```python
from build123d import *

# Parameters (mm, degrees)
SZKIC1_W                    = 140
SZKIC1_H                    = 70
DODANIE_WYCI_GNI_CIE1_DEPTH = 5
SZKIC2_W                    = 4
SZKIC2_H                    = 30
DODANIE_WYCI_GNI_CIE2_DEPTH = 25
SZKIC3_W                    = 10
SZKIC3_H                    = 30
SZKIC3_W_2                  = 2
DODANIE_WYCI_GNI_CIE3_DEPTH = 2
SZKIC4_R                    = 0.75
WYTNIJ_WYCI_GNI_CIE1_DEPTH  = 12
WYTNIJ_WYCI_GNI_CIE2_START  = -12
SZKIC5_R                    = 0.75
WYTNIJ_WYCI_GNI_CIE2_DEPTH  = 12
SZKIC6_W                    = 5
SZKIC6_H                    = 20
WYTNIJ_WYCI_GNI_CIE3_DEPTH  = 12
SZKIC8_R                    = 1
WYTNIJ_WYCI_GNI_CIE4_DEPTH  = 12


with BuildPart() as part:
    # Szkic1 → Dodanie-wyciągnięcie1 (new body)
    with BuildSketch(Plane(origin=(0, 0, 0), x_dir=(1, 0, 0), z_dir=(0, 1, 0))):
        with Locations((70, -35)):
            Rectangle(SZKIC1_W, SZKIC1_H)
    extrude(amount=DODANIE_WYCI_GNI_CIE1_DEPTH)

    # Szkic2 → Dodanie-wyciągnięcie2 (add)
    with BuildSketch(Plane.XZ):
        with Locations((2, 35)):
            Rectangle(SZKIC2_W, SZKIC2_H)
        with Locations((138, 35)):
            Rectangle(SZKIC2_W, SZKIC2_H)
        with Locations((70, 35)):
            Rectangle(SZKIC2_W, SZKIC2_H)
    extrude(amount=DODANIE_WYCI_GNI_CIE2_DEPTH)

    # Szkic3 → Dodanie-wyciągnięcie3 (add)
    with BuildSketch(Plane.XZ.offset(25)):
        with Locations((77, 35)):
            Rectangle(SZKIC3_W, SZKIC3_H)
        with Locations((63, 35)):
            Rectangle(SZKIC3_W, SZKIC3_H)
        with Locations((71, 35)):
            Rectangle(SZKIC3_W_2, SZKIC3_H)
        with Locations((69, 35)):
            Rectangle(SZKIC3_W_2, SZKIC3_H)
    extrude(amount=DODANIE_WYCI_GNI_CIE3_DEPTH)

    # Szkic4 → Wytnij-wyciągnięcie1 (cut)
    with BuildSketch(Plane.ZY):
        with Locations((35, -2.75)):
            Circle(SZKIC4_R)
        with Locations((35, -21.25)):
            Circle(SZKIC4_R)
    extrude(amount=-WYTNIJ_WYCI_GNI_CIE1_DEPTH, mode=Mode.SUBTRACT)

    # Szkic5 → Wytnij-wyciągnięcie2 (cut)
    with BuildSketch(Plane(origin=(140, 0, 0), x_dir=(0, 0, -1), z_dir=(1, 0, 0)).offset(WYTNIJ_WYCI_GNI_CIE2_START)):
        with Locations(Location((-35, -21.25, 0), (0, 0, 180))):
            Circle(SZKIC5_R)
        with Locations(Location((-35, -2.75, 0), (0, 0, 180))):
            Circle(SZKIC5_R)
    extrude(amount=WYTNIJ_WYCI_GNI_CIE2_DEPTH, mode=Mode.SUBTRACT)

    # Szkic6 → Wytnij-wyciągnięcie3 (cut)
    with BuildSketch(Plane(origin=(0, 5, 0), x_dir=(1, 0, 0), z_dir=(0, 1, 0))):
        with Locations((58.5, -35)):
            Rectangle(SZKIC6_W, SZKIC6_H)
        with Locations((81.5, -35)):
            Rectangle(SZKIC6_W, SZKIC6_H)
    extrude(amount=-WYTNIJ_WYCI_GNI_CIE3_DEPTH, mode=Mode.SUBTRACT)

    # Szkic8 → Wytnij-wyciągnięcie4 (cut)
    with BuildSketch(Plane(origin=(0, 5, 0), x_dir=(1, 0, 0), z_dir=(0, 1, 0))):
        with Locations(Location((135, -65, 0), (0, 0, 270))):
            Circle(SZKIC8_R)
        with Locations(Location((135, -5, 0), (0, 0, 270))):
            Circle(SZKIC8_R)
        with Locations(Location((5, -5, 0), (0, 0, 270))):
            Circle(SZKIC8_R)
        with Locations(Location((5, -65, 0), (0, 0, 270))):
            Circle(SZKIC8_R)
    extrude(amount=-WYTNIJ_WYCI_GNI_CIE4_DEPTH, mode=Mode.SUBTRACT)


solid = part.part
```
CAD build for the part. Positions are in the model's coordinates, mm. A direction names the side the tool comes from. Round coordinates to 2 decimals unless told otherwise and drop trailing zeros. Loops run counter-clockwise (first coordinate to the right, second up) from the corner with the lowest first, then second, coordinate; pieces in that order, holes last. Notation, with made-up numbers: (-31.5, 68) - (16.5, 68) arc R19 ccw to (16.5, 77) - close; hole circle Ø11 at (-37.75, 57.5). An arc over 180 degrees is marked (long way). Return JSON: item names as keys, results as strings. Group by question number.
Q1. Flat gauge pins, fed straight in: pin 1 Ø12 at (x, y) = (56.5, -21.5) entering from -Z; pin 2 Ø1.6 at (x, z) = (5, 5) entering from +Y; pin 3 Ø4.5 at (x, y) = (137.5, -7) entering from +Z; pin 4 Ø10 at (x, z) = (97, 52) entering from -Y. Where does each tip first touch, or does it go through?
Q2. Tool access for faces 4 (the face through (61, 3, 35)), 5 (the face through (138, -12, 20)), 6 (the face through (63, -25, 35)), 7 (the face through (56, 3, 35)): list every direction of +Z, -Z, +X, -X, +Y, -Y with a clear straight run to the whole face (end or side of a thin tool).
Q3. Two-plate mould, pull along X, no slides. Class faces 1 (the face through (70, -27, 35)), 2 (the face through (58, 3, 45)), 3 (the face through (0, -7, 35)): +X half, -X half, draft (parallel to the pull), parting line (faces both ways), or undercut.
Q4. Band-saw the part on D-D on z = 59.5. Give the cut face in (x, y).
Q5. Drill centre lines: line 1 along X through (y, z) = (-3.5, 45.5); line 2 along X through (y, z) = (1.45, 65); line 3 along Y through (x, z) = (138.35, 35). Where is each one in solid material? Low to high. Write a range as [from, to].
Q6. Band-saw the part on A-A on y = -19. Give the cut face in (x, z), plus the area to 3 significant figures.
Q7. Band-saw the part on B-B on z = 23. Give the cut face in (x, y), plus the area to 3 significant figures.
Q8. Band-saw the part on C-C on x = 19. Give the cut face in (y, z), plus the area to 3 significant figures.
Solutions:
{
 "1": {"pin 1": "stops at z = 20", "pin 2": "passes through", "pin 3": "stops at z = 50", "pin 4": "stops at y = 0"},
 "2": {"face 4": "+Y", "face 5": "-Z, +X, -X, -Y", "face 6": "+Z, -Z", "face 7": "+Y, -Y"},
 "3": {"face 1": "draft", "face 2": "undercut", "face 3": "-X half"},
 "4": {"outline": "(0, 0) - (140, 0) - (140, 5) - (0, 5) - close"},
 "5": {"line 1": "x = [0, 4], [68, 72], [136, 140]", "line 2": "x = [0, 4], [6, 134], [136, 140]", "line 3": "y = [-25, -22], [-20.5, -3.5], [-2, 5]"},
 "6": {"outline": "(0, 20) - (4, 20) - (4, 50) - (0, 50) - close; (68, 20) - (72, 20) - (72, 50) - (68, 50) - close; (136, 20) - (140, 20) - (140, 50) - (136, 50) - close", "area": "360 mm^2"},
 "7": {"outline": "(0, -25) - (4, -25) - (4, 0) - (68, 0) - (68, -25) - (58, -25) - (58, -27) - (82, -27) - (82, -25) - (72, -25) - (72, 0) - (136, 0) - (136, -25) - (140, -25) - (140, 5) - (0, 5) - close", "area": "1,050 mm^2"},
 "8": {"outline": "(0, 0) - (5, 0) - (5, 70) - (0, 70) - close", "area": "350 mm^2"}
}
